from build123d import *

# Parameters (mm, degrees)
F0_R     = 2.04
F1_DEPTH = 1.4
F2_W     = 10.66
F2_H     = 9.66
F3_DEPTH = 3.42
F4_W     = 1.77
F4_H     = 0.5
F5_DEPTH = 6.35
F6_W     = 1.01
F6_H     = 0.5
F7_DEPTH = 3


with BuildPart() as f1:
    # F0 (on Front) → F1 (new body)
    with BuildSketch(Plane.XZ):
        Polygon((5.33, 16.51), (-5.33, 16.51), (-5.33, 14.89), (-4.53, 14.89), (-4.53, 13.09), (-5.33, 13.09), (-5.33, 0), (5.33, 0), (5.33, 13.09), (4.53, 13.09), (4.53, 14.89), (5.33, 14.89), align=None)
        with Locations((0, 13.09)):
            Circle(F0_R, mode=Mode.SUBTRACT)
    extrude(amount=-F1_DEPTH)

    # F2 (on face) → F3 (join)
    with BuildSketch(Plane.XZ):
        with Locations((0, 4.83)):
            Rectangle(F2_W, F2_H)
    extrude(amount=F3_DEPTH)

    # F4 (on face) → F5 (join)
    with BuildSketch(Plane(origin=(0, 0, 0), x_dir=(1, 0, 0), z_dir=(0, 0, -1))):
        with Locations((-2.79, 1.77)):
            Rectangle(F4_W, F4_H)
        with Locations((0, 1.77)):
            Rectangle(F4_W, F4_H)
        with Locations((2.79, 1.77)):
            Rectangle(F4_W, F4_H)
    extrude(amount=F5_DEPTH)

    # F6 (on face) → F7 (join)
    with BuildSketch(Plane(origin=(0, 0, -6.35), x_dir=(1, 0, 0), z_dir=(0, 0, -1))):
        with Locations((-2.79, 1.77)):
            Rectangle(F6_W, F6_H)
        with Locations((0, 1.77)):
            Rectangle(F6_W, F6_H)
        with Locations((2.79, 1.77)):
            Rectangle(F6_W, F6_H)
    extrude(amount=F7_DEPTH)


solid = f1.part
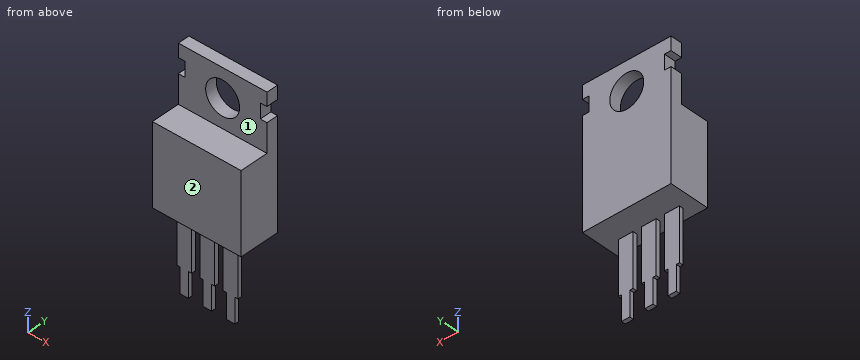
For this review, take the finished solid that the model builds, in its own axes (mm). Face numbers are marked on the shaded views. A direction names the side the tool comes from. Coordinates: 2 decimals unless noted, no trailing zeros. Order: outer loops, then holes, each group sorted by start corner. A loop starts at its lowest first (then second) coordinate and runs counter-clockwise, first axis right, second up. Notation, with made-up numbers: (-12, 18) - (19, 18) arc R25 ccw to (19, 31) - close; hole circle Ø4 at (27.5, 49). An arc over 180 degrees is marked (long way). Answer as CSV lines item,"result". Start each with the question number.
1) Add section A-A (x = 0). State the section outline as (y, z) points, then the cut area to 3 significant figures.
2) Machinability: for the marked faces 1 and 2, which of the approach directions +Z, -Z, +X, -X, +Y, -Y give a long, thin tool a straight path to every point of the face, cutting with its end or side? Answer none if there is none.
3) Insertion check: P1, Ø0.9, axis at x = -3, z = -7, coming from the +Y side; P2, Ø0.6, axis at y = -2, z = -8.5, coming from the +X side (3 decimals); P3, Ø1, axis at x = -2.5, z = -3, coming from the -Y side. Each pin has a flat end and moves straight along its axis. Give the tip position at first contact, or say it passes through.
4) Add section D-D (z = 10). State the section outline as (x, y) points.
5) To check wall thickness, follow line 1 along Z through (x, y) = (0, 0.4); line 2 along Z through (x, y) = (-2.25, 0.6); line 3 along Y through (x, z) = (3, 13.75). State the ranges of each line that lie inside material, in increasing order. Write a range as [from, to].
6) Add section C-C (x = -1.25). State the section outline as (y, z) points.
7) Add section B-B (y = 0.9). State the section outline as (x, z) points, then the cut area to 3 significant figures.
Result:
1,outline,"(-3.42, 0) - (-2.02, 0) - (-2.02, -9.35) - (-1.52, -9.35) - (-1.52, 0) - (1.4, 0) - (1.4, 11.05) - (0, 11.05) - (0, 9.66) - (-3.42, 9.66) - close; (0, 15.13) - (1.4, 15.13) - (1.4, 16.51) - (0, 16.51) - close"
1,area,"55.1 mm^2"
2,face 1,"+Z, +X, -X, -Y"
2,face 2,"+Z, -Z, +X, -X, -Y"
3,P1,"y = -1.52"
3,P2,"x = 3.295"
3,P3,"y = -2.02"
4,outline,"(-5.33, 0) - (5.33, 0) - (5.33, 1.4) - (-5.33, 1.4) - close"
5,line 1,"[0, 11.05], [15.13, 16.51]"
5,line 2,"[0, 16.51]"
5,line 3,"[0, 1.4]"
6,outline,"(-3.42, 0) - (1.4, 0) - (1.4, 11.48) - (0, 11.48) - (0, 9.66) - (-3.42, 9.66) - close; (0, 14.7) - (1.4, 14.7) - (1.4, 16.51) - (0, 16.51) - close"
7,outline,"(-5.33, 0) - (5.33, 0) - (5.33, 13.09) - (4.53, 13.09) - (4.53, 14.89) - (5.33, 14.89) - (5.33, 16.51) - (-5.33, 16.51) - (-5.33, 14.89) - (-4.53, 14.89) - (-4.53, 13.09) - (-5.33, 13.09) - close; hole circle Ø4.08 at (0, 13.09)"
7,area,"160 mm^2"
